Can you work these out from the model? Positions are in its coordinate system, mm. A direction names the side the tool comes from. Give positions to 0.01 mm unless a question says otherwise; leave off trailing zeros. Write each loop counter-clockwise with the first axis right and the second up, starting at its lowest first coordinate (ties: lowest second). Pieces come first, ordered by that corner, then holes. Notation, with made-up numbers: (59.25, 6) -> (69.25, 6) arc R33 cw to (69.25, 36) -> close; hole circle Ø1 at (10, -34). An arc over 180 degrees is marked (long way). Answer as CSV lines item,"result". Start each with the question number.
1. If we section it at C-C on y = 2.25: Write out the boundary of the cut face in (x, z), plus the area to 3 significant figures.
2. On a 3-axis mill with a long thin cutter (end or side, diameter ignored), from which of +Z, -Z, +X, -X, +Y, -Y can I reach the whole of each face in a straight line? I mean faces 1 (the face through (3, 0, -3.8)), 2 (the face through (3, 1, -3.5)), 3 (the face through (3, 3.1, 0)). Say none if no direction works.
3. I'm going to push flat-ended pins straight in: P1, Ø1.1, axis at x = 3.5, y = -0.5, coming from the -Z side; P2, Ø0.7, axis at x = 3, y = -0.5, coming from the +Z side; P3, Ø5, axis at x = 2, z = -0.5, coming from the +Y side. Where does each tip first touch, or does it pass through?
4. If we section it at B-B on z = 0.5: Write out the boundary of the cut face in (x, y), plus the area to 3 significant figures.
5. If we section it at D-D on z = -1.5: Write out the boundary of the cut face in (x, y).
6. I need wall thicknesses on line 1 (Y direction, x = 4.5, z = -2.25); line 2 (Y direction, x = 1.25, z = 1); line 3 (Z direction, x = 2.5, y = -1.75). Which ranges of each line are inside material? Lowest first, please. Write a range as [from, to].
7. If we mould it in two halves opening along Z, with no side actions, what happens to faces 4 (the face through (2.6, -2.3, -3)), 5 (the face through (0, 0, 0)), 6 (the face through (2.6, -2.3, 3)), 7 (the face through (5.86, -2.72, 3.4))? For each: pulls with the +Z half, pulls with the -Z half, needs draft (parallel to the pull), parting line crosses it, or undercut.
8. If we section it at A-A on y = 0.25: Write out the boundary of the cut face in (x, z), plus the area to 3 significant figures.
```python
from build123d import *

# Parameters (mm, degrees)
BOSS_EXTRUDE1_DEPTH = 5
BOSS_EXTRUDE2_DEPTH = 5
CHAMFER1_SIZE       = 0.3
CHAMFER2_SIZE       = 0.2
BOSS_EXTRUDE3_DEPTH = 1
BOSS_EXTRUDE4_DEPTH = 0.6
CHAMFER4_SIZE       = 0.2
SKETCH5_W           = 10
SKETCH5_H           = 10
BOSS_EXTRUDE5_DEPTH = 5
FILLET1_R           = 0.5


with BuildPart() as part:
    # Sketch1 → Boss-Extrude1 (new body)
    with BuildSketch(Plane(origin=(0, 0, 0), x_dir=(0, 0, -1), z_dir=(1, 0, 0))):
        with BuildLine():
            Line((-2.2, 1), (2.2, 1))
            ThreePointArc((2.2, 1), (2.412132034, 0.912132034), (2.5, 0.7))
            Line((2.5, 0.7), (2.5, -0.7))
            ThreePointArc((2.5, -0.7), (2.412132034, -0.912132034), (2.2, -1))
            Line((2.2, -1), (-2.2, -1))
            ThreePointArc((-2.2, -1), (-2.412132034, -0.912132034), (-2.5, -0.7))
            Line((-2.5, -0.7), (-2.5, 0.7))
            ThreePointArc((-2.5, 0.7), (-2.412132034, 0.912132034), (-2.2, 1))
        make_face()
    extrude(amount=BOSS_EXTRUDE1_DEPTH)

    # Chamfer1
    chamfer1_edges = [part.edges().sort_by_distance(p)[0] for p in [
        (0, -1, 0),
        (0, -0.912132034, 2.412132034),
        (0, 0, 2.5),
        (0, 0.912132034, 2.412132034),
        (0, 1, 0),
        (0, 0.912132034, -2.412132034),
        (0, 0, -2.5),
        (0, -0.912132034, -2.412132034),
    ]]
    chamfer(chamfer1_edges, length=CHAMFER1_SIZE - 0.0001)  # a hair under: the kernel refuses the full size



with BuildPart() as body_2:
    # Sketch2 → Boss-Extrude2 (new body)
    with BuildSketch(Plane.ZY):
        Polygon((3.8, -2.1), (2.8, -3.1), (-2.8, -3.1), (-3.8, -2.1), (-3.8, 3.1), (3.8, 3.1), align=None)
        Polygon((3.5, 2.8), (-3.5, 2.8), (-3.5, -1.8), (-2.5, -2.8), (2.5, -2.8), (3.5, -1.8), align=None, mode=Mode.SUBTRACT)
    extrude(amount=-BOSS_EXTRUDE2_DEPTH)

    # Chamfer2
    chamfer2_edges = [body_2.edges().sort_by_distance(p)[0] for p in [
        (0, 0.5, 3.5),
        (0, 2.8, 0),
        (0, 0.5, -3.5),
        (0, -2.3, -3),
        (0, -2.8, 0),
        (0, -2.3, 3),
    ]]
    chamfer(chamfer2_edges, length=CHAMFER2_SIZE)


with BuildPart() as part_1:
    add(part.part)

    add(body_2.part)  # Boss-Extrude3 merges body 2
    # Sketch3 → Boss-Extrude3 (add)
    with BuildSketch(Plane(origin=(5, 0, 0), x_dir=(0, 0, -1), z_dir=(1, 0, 0))):
        Polygon((-3.8, -2.1), (-2.8, -3.1), (2.8, -3.1), (3.8, -2.1), (3.8, 3.1), (-3.8, 3.1), align=None)
    extrude(amount=BOSS_EXTRUDE3_DEPTH)

    # Sketch4 → Boss-Extrude4 (add)
    with BuildSketch(Plane.XZ.offset(3.1)):
        with BuildLine():
            Line((1, 0.8), (1, -0.8))
            ThreePointArc((1, -0.8), (1.527586443, -1.327586443), (2.055172886, -0.8))
            Line((2.055172886, -0.8), (2.055172886, 0.8))
            ThreePointArc((2.055172886, 0.8), (1.527586443, 1.327586443), (1, 0.8))
        make_face()
    extrude(amount=-BOSS_EXTRUDE4_DEPTH)

    # Chamfer4
    chamfer4_edges = [part_1.edges().sort_by_distance(p)[0] for p in [
        (1.527586443, -2.5, 1.327586443),
        (2.055172886, -2.5, 0),
        (1.527586443, -2.5, -1.327586443),
        (1, -2.5, 0),
    ]]
    chamfer(chamfer4_edges, length=CHAMFER4_SIZE)

    # Sketch5 → Boss-Extrude5 (add)
    with BuildSketch(Plane(origin=(6, 0, 0), x_dir=(0, 0, -1), z_dir=(1, 0, 0))):
        with Locations((0, 0.5)):
            Rectangle(SKETCH5_W, SKETCH5_H)
    extrude(amount=BOSS_EXTRUDE5_DEPTH)

    # Fillet1
    fillet1_edges = [part_1.edges().sort_by_distance(p)[0] for p in [
        (6, 0.5, 3.8),
        (6, -2.6, 3.3),
        (6, -3.1, 0),
        (6, -2.6, -3.3),
        (6, 0.5, -3.8),
        (6, 3.1, 0),
    ]]
    fillet(fillet1_edges, radius=FILLET1_R)


solid = part_1.part
```
Computed values:
1,outline,"(0, -3.8) -> (5.5, -3.8) arc R0.5 cw to (6, -4.3) -> (6, -5) -> (11, -5) -> (11, 5) -> (6, 5) -> (6, 4.3) arc R0.5 cw to (5.5, 3.8) -> (0, 3.8) -> (0, 3.7) -> (0.2, 3.5) -> (5, 3.5) -> (5, -3.5) -> (0.2, -3.5) -> (0, -3.7) -> close"
1,area,"60.7 mm2"
2,face 1,"-Z, -X, +Y, -Y"
2,face 2,"-X"
2,face 3,"+Z, -Z, -X, +Y"
3,P1,"stops at z = -3.8"
3,P2,"stops at z = 3.8"
3,P3,"stops at y = 3.1"
4,outline,"(0, -3.1) -> (5.5, -3.1) arc R0.5 cw to (6, -3.6) -> (6, -4.5) -> (11, -4.5) -> (11, 5.5) -> (6, 5.5) -> (6, 3.6) arc R0.5 cw to (5.5, 3.1) -> (0, 3.1) -> (0, 3) -> (0.2, 2.8) -> (5, 2.8) -> (5, 1) -> (0.3, 1) -> (0, 0.7) -> (0, -0.7) -> (0.3, -1) -> (5, -1) -> (5, -2.8) -> (2.06, -2.8) -> (2.06, -2.7) -> (1.86, -2.5) -> (1.2, -2.5) -> (1, -2.7) -> (1, -2.8) -> (0.2, -2.8) -> (0, -3) -> close"
4,area,"69.5 mm2"
5,outline,"(0, -3.1) -> (5.5, -3.1) arc R0.5 cw to (6, -3.6) -> (6, -4.5) -> (11, -4.5) -> (11, 5.5) -> (6, 5.5) -> (6, 3.6) arc R0.5 cw to (5.5, 3.1) -> (0, 3.1) -> (0, 3) -> (0.2, 2.8) -> (5, 2.8) -> (5, 1) -> (0.3, 1) -> (0, 0.7) -> (0, -0.7) -> (0.3, -1) -> (5, -1) -> (5, -2.8) -> (0.2, -2.8) -> (0, -3) -> close"
6,line 1,"y = [-3.1, -2.8], [-1, 1], [2.8, 3.1]"
6,line 2,"y = [-3.1, -2.51], [-1, 1], [2.8, 3.1]"
6,line 3,"z = [-3.8, -3.5], [3.5, 3.8]"
7,face 4,"undercut"
7,face 5,"needs draft"
7,face 6,"undercut"
7,face 7,"pulls with the +Z half"
8,outline,"(0, -3.8) -> (5.5, -3.8) arc R0.5 cw to (6, -4.3) -> (6, -5) -> (11, -5) -> (11, 5) -> (6, 5) -> (6, 4.3) arc R0.5 cw to (5.5, 3.8) -> (0, 3.8) -> (0, 3.7) -> (0.2, 3.5) -> (5, 3.5) -> (5, 2.5) -> (0.3, 2.5) -> (0, 2.2) -> (0, -2.2) -> (0.3, -2.5) -> (5, -2.5) -> (5, -3.5) -> (0.2, -3.5) -> (0, -3.7) -> close"
8,area,"85.6 mm2"
